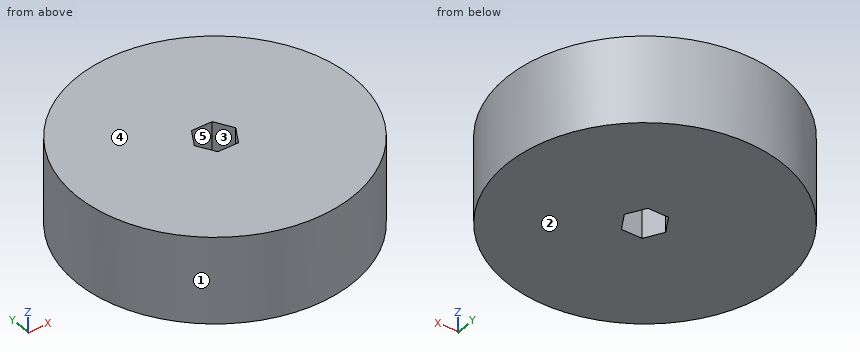
```python
from build123d import *

# Parameters (mm, degrees)
SKETCH1_R           = 24
BOSS_EXTRUDE1_DEPTH = 15
CUT_EXTRUDE1_DEPTH  = 38.107950631
SCALE1_SCALE        = 0.75


with BuildPart() as part:
    # Sketch1 → Boss-Extrude1 (new body)
    with BuildSketch(Plane.XY):
        Circle(SKETCH1_R)
    extrude(amount=BOSS_EXTRUDE1_DEPTH)

    # Sketch2 → Cut-Extrude1 (cut, through all)
    with BuildSketch(Plane.XY.offset(15)):
        Polygon((3.6, 0), (1.8, 3.117691454), (-1.8, 3.117691454), (-3.6, 0), (-1.8, -3.117691454), (1.8, -3.117691454), align=None)
    extrude(amount=-CUT_EXTRUDE1_DEPTH, mode=Mode.SUBTRACT)


with BuildPart() as part_1:
    # Scale1: scaled about (0, 0, 7.5)
    add(part.part.scale(SCALE1_SCALE).moved(Location((0, 0, 1.875))))


solid = part_1.part
```
Can you work these out from the model? Positions are in its coordinate system, mm. Face numbers are marked on the shaded views. A direction names the side the tool comes from. Give positions to 0.01 mm unless a question says otherwise; leave off trailing zeros. Write each loop counter-clockwise with the first axis right and the second up, starting at its lowest first coordinate (ties: lowest second). Pieces come first, ordered by that corner, then holes. Notation, with made-up numbers: (22.5, -16) - (26.5, -16) arc R17 ccw to (26.5, -2) - close; hole circle Ø9 at (73, 73.5). An arc over 180 degrees is marked (long way). Write item = value, one per line. Start each with the question number.
1. Imagine slicing it at D-D (y = 13). Please give me the cut outline in (x, z) (3 decimals).
2. Imagine slicing it at B-B (z = 4). Please give me the cut outline in (x, y).
3. For pin 1 (3 mm diameter, centred on x = 0.5, z = 9.5, fed in from +Y); pin 2 (5 mm diameter, centred on y = -5, z = 7.5, fed in from +X); pin 3 (6 mm diameter, centred on y = 7.5, z = 5.5, fed in from +X), each with a flat end and sliding along its axis, tell me the tip position at first contact or that it passes through.
4. Imagine slicing it at C-C (y = -1). Please give me the cut outline in (x, z) (3 decimals), and give its area (3 significant figures).
5. Imagine slicing it at A-A (x = 0). Please give me the cut outline in (y, z) (3 decimals), and give its area (3 significant figures).
6. On a 3-axis mill with a long thin cutter (end or side, diameter ignored), from which of +Z, -Z, +X, -X, +Y, -Y can I reach the whole of each face in a straight line? I mean the marked faces 4 and 5. Say none if no direction works.
7. Thinking about a two-plate mould opening in Y: for the marked faces 1, 2 and 3, which applies, released by +Y, released by -Y, zero draft, split by the parting line, or undercut?
8. Please list where these lines run through material, in increasing order: line 1 (Y direction, x = -0.5, z = 4.5); line 2 (X direction, y = -10, z = 8.75); line 3 (Y direction, x = -9, z = 5).
Worked answers:
q1.outline = (-12.45, 1.875) - (12.45, 1.875) - (12.45, 13.125) - (-12.45, 13.125) - close
q2.outline = circle Ø36 at (0, 0); hole (-2.7, 0) - (-1.35, -2.34) - (1.35, -2.34) - (2.7, 0) - (1.35, 2.34) - (-1.35, 2.34) - close
q3.pin_1 = 18
q3.pin_2 = 17.83
q3.pin_3 = 17.43
q4.outline = (-17.972, 1.875) - (-2.123, 1.875) - (-2.123, 13.125) - (-17.972, 13.125) - close; (2.123, 1.875) - (17.972, 1.875) - (17.972, 13.125) - (2.123, 13.125) - close
q4.area = 357 mm2
q5.outline = (-18, 1.875) - (-2.338, 1.875) - (-2.338, 13.125) - (-18, 13.125) - close; (2.338, 1.875) - (18, 1.875) - (18, 13.125) - (2.338, 13.125) - close
q5.area = 352 mm2
q6.face_4 = +Z, +X, -X, +Y, -Y
q6.face_5 = +Z, -Z
q7.face_1 = split by the parting line
q7.face_2 = zero draft
q7.face_3 = undercut
q8.line_1 = -17.99 to -2.34, 2.34 to 17.99
q8.line_2 = -14.97 to 14.97
q8.line_3 = -15.59 to 15.59
